from build123d import *

# Parameters (mm, degrees)
SKETCH1_R           = 2.075
SKETCH1_R_2         = 6.003208263
BOSS_EXTRUDE2_DEPTH = 8
FILLET1_R           = 2


with BuildPart() as part:
    # Sketch1 → Boss-Extrude2 (new body)
    with BuildSketch(Plane(origin=(0, 0, 0), x_dir=(1, 0, 0), z_dir=(0, 1, 0))):
        with BuildLine():
            Line((0, 44.83), (0, 36.83))
            ThreePointArc((0, 36.83), (36.83, 0), (0, -36.83))
            Line((0, -36.83), (0, -46.83))
            Line((0, -46.83), (0, -58.83))
            ThreePointArc((0, -58.83), (14.116701064, -87.229775601), (8, -56.110417137))
            Line((8, -56.110417137), (8, -44.110417137))
            ThreePointArc((8, -44.110417137), (44.649741882, 4.016148637), (0, 44.83))
        make_face()
        with Locations(Location((0.96696537, -64.081170969, 0), (0, 0, 270))):
            Circle(SKETCH1_R, mode=Mode.SUBTRACT)
        with Locations(Location((16.96696537, -64.081170969, 0), (0, 0, 270))):
            Circle(SKETCH1_R, mode=Mode.SUBTRACT)
        with Locations(Location((16.96696537, -80.081170969, 0), (0, 0, 270))):
            Circle(SKETCH1_R, mode=Mode.SUBTRACT)
        with Locations(Location((0.96696537, -80.081170969, 0), (0, 0, 270))):
            Circle(SKETCH1_R, mode=Mode.SUBTRACT)
        with Locations(Location((8.96696537, -72.081170969, 0), (0, 0, 270))):
            Circle(SKETCH1_R_2, mode=Mode.SUBTRACT)
    extrude(amount=BOSS_EXTRUDE2_DEPTH)

    # Fillet1
    fillet1_edges = [part.edges().sort_by_distance(p)[0] for p in [
        (0, 4, 58.83),
        (0, 4, 36.83),
        (0, 4, -36.83),
        (0, 4, -44.83),
        (8, 4, 44.110417137),
        (8, 4, 56.110417137),
    ]]
    fillet(fillet1_edges, radius=FILLET1_R)


solid = part.part
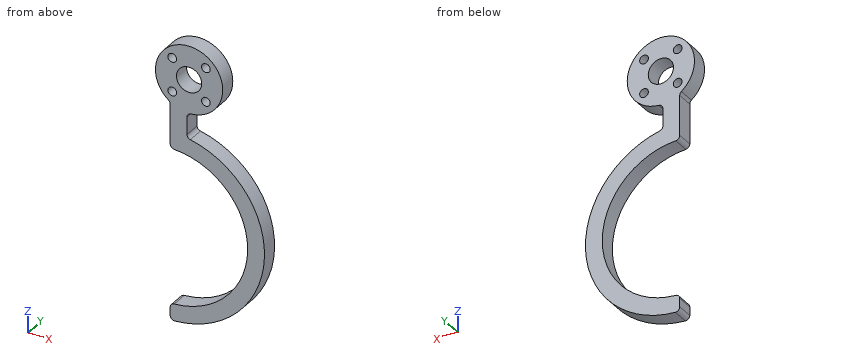
Could you check a few things on this model? Use its own coordinates, in mm. Coordinates: 2 decimals unless noted, no trailing zeros. Order: outer loops, then holes, each group sorted by start corner. A loop starts at its lowest first (then second) coordinate and runs counter-clockwise, first axis right, second up.
Q1. Please list where these lines run through material, in increasing order: L1, parallel to Z at x = 7, y = 4; L2, parallel to Z at x = 11.5, y = 1; L3, parallel to Z at x = 14, y = 3.75.
Q2. Will these pins go through, and if not, where does the flat tip stop? pin 1 (2 mm diameter, centred on y = 3.5, z = -40, fed in from -X); pin 2 (1 mm diameter, centred on y = 3, z = 26.5, fed in from +X); pin 3 (3.5 mm diameter, centred on x = 0.97, z = 80.08, fed in from -Y); pin 4 (1.5 mm diameter, centred on x = 4.5, y = 2, fed in from +Z).
Q3. Suppose I cut it at B-B on y = 3. Please give me the cut outline in (x, z) (3 decimals).
Q4. Suppose I cut it at A-A on x = 4.5. Please give me the cut outline in (y, z), and give its area (3 significant figures).
Q5. Suppose I cut it at C-C on x = 28. Please give me the cut outline in (y, z).
Q6. Suppose I cut it at D-D on z = 0. Please give me the cut outline in (x, y), and give its area (3 significant figures).
Answer:
1. L1: z = -44.28 to -36.16, 36.16 to 66.41, 77.75 to 87.96
1. L2: z = -43.33 to -34.99, 34.99 to 43.33, 56.28 to 66.64, 77.52 to 87.88
1. L3: z = -42.59 to -34.07, 34.07 to 42.59, 56.89 to 68.81, 75.35 to 87.27
2. pin 1: stops at x = 0
2. pin 2: stops at x = 36.52
2. pin 3: passes through
2. pin 4: stops at z = 87.64
3. outline: (-0.781, 59.394) arc R2 cw to (0, 57.808) - (0, 38.778) arc R2 ccw to (1.897, 36.781) arc R36.83 cw to (1.897, -36.781) arc R2 ccw to (0, -38.778) - (0, -42.783) arc R2 ccw to (2.093, -44.781) arc R44.83 ccw to (9.573, 43.796) arc R2 cw to (8, 45.75) - (8, 54.111) arc R2 cw to (9.885, 56.108) arc R16 ccw (long way) to start; hole circle Ø4.15 at (0.967, 64.081); hole circle Ø4.15 at (0.967, 80.081); hole circle Ø12.006 at (8.967, 72.081); hole circle Ø4.15 at (16.967, 64.081); hole circle Ø4.15 at (16.967, 80.081)
4. outline: (0, -44.6) - (8, -44.6) - (8, -36.55) - (0, -36.55) - close; (0, 36.55) - (8, 36.55) - (8, 68.07) - (0, 68.07) - close; (0, 76.09) - (8, 76.09) - (8, 87.44) - (0, 87.44) - close
4. area: 407 mm2
5. outline: (0, -35.01) - (8, -35.01) - (8, -23.93) - (0, -23.93) - close; (0, 23.93) - (8, 23.93) - (8, 35.01) - (0, 35.01) - close
6. outline: (36.83, 0) - (44.83, 0) - (44.83, 8) - (36.83, 8) - close
6. area: 64.0 mm2
